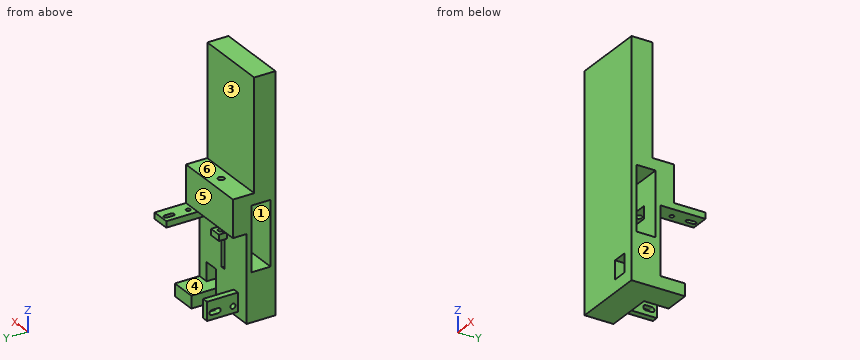
```python
from build123d import *

# Parameters (mm, degrees)
SKETCH1_W               = 60
SKETCH1_H               = 70
BOSS_EXTRUDE1_DEPTH     = 23.5
SHELL1_T                = -9
SKETCH2_W               = 10
SKETCH2_H               = 5
BOSS_EXTRUDE2_DEPTH     = 6.5
SKETCH5_W               = 60
SKETCH5_H               = 30
BOSS_EXTRUDE3_DEPTH     = 11
CUT_EXTRUDE1_DEPTH      = 83.554527435
CUT_EXTRUDE1_DEPTH_BACK = 83.554527435
SKETCH3_R               = 2.5
SKETCH4_W               = 30
SKETCH4_H               = 10
CUT_EXTRUDE2_DEPTH      = 10
SKETCH6_W               = 15
SKETCH6_H               = 5
BOSS_EXTRUDE4_DEPTH     = 36.5
SKETCH8_R               = 1.75
CUT_EXTRUDE3_DEPTH      = 10
SKETCH9_W               = 60
SKETCH9_H               = 23.5
BOSS_EXTRUDE5_DEPTH     = 30
CUT_EXTRUDE4_DEPTH      = 123.197585901
CUT_EXTRUDE4_DEPTH_BACK = 123.197585901
SKETCH11_W              = 12
SKETCH11_H              = 15
SKETCH12_W              = 5
SKETCH12_H              = 15
BOSS_EXTRUDE7_DEPTH     = 25
SKETCH13_R              = 2
CUT_EXTRUDE5_DEPTH      = 25
SKETCH14_W              = 21
SKETCH14_H              = 10
BOSS_EXTRUDE8_DEPTH     = 20
SKETCH15_W              = 60
SKETCH15_H              = 17.25
BOSS_EXTRUDE9_DEPTH     = 90
CUT_EXTRUDE6_DEPTH      = 132.148770486
CUT_EXTRUDE6_DEPTH_BACK = 132.148770486
SKETCH16_W              = 52
SKETCH16_H              = 15.5


with BuildPart() as part:
    # Sketch1 → Boss-Extrude1 (new body)
    with BuildSketch(Plane(origin=(0, 0, 0), x_dir=(1, 0, 0), z_dir=(0, 1, 0))):
        with Locations((-30, 35)):
            Rectangle(SKETCH1_W, SKETCH1_H)
    extrude(amount=BOSS_EXTRUDE1_DEPTH)

    # Shell1
    shell1_openings = [part.faces().sort_by_distance(p)[0] for p in [
        (-60, 11.75, -35),
        (0, 11.75, -35),
    ]]
    offset(amount=SHELL1_T, openings=shell1_openings, kind=Kind.INTERSECTION)

    # Sketch2 → Boss-Extrude2 (add)
    with BuildSketch(Plane(origin=(0, 23.5, 0), x_dir=(1, 0, 0), z_dir=(0, 1, 0))):
        with Locations((-30, 42.5)):
            Rectangle(SKETCH2_W, SKETCH2_H)
        with Locations((-30, 27.5)):
            Rectangle(SKETCH2_W, SKETCH2_H)
    extrude(amount=BOSS_EXTRUDE2_DEPTH)

    # Sketch5 → Boss-Extrude3 (add)
    with BuildSketch(Plane(origin=(0, 23.5, 0), x_dir=(1, 0, 0), z_dir=(0, 1, 0))):
        with Locations((-30, 15)):
            Rectangle(SKETCH5_W, SKETCH5_H)
    extrude(amount=BOSS_EXTRUDE3_DEPTH)

    # Sketch3 → Cut-Extrude1 (cut, two sides: drawn at the far end of the back side and taken through both)
    with BuildSketch(Plane(origin=(0, 0, -45), x_dir=(-1, 0, 0), z_dir=(0, 0, -1)).offset(-CUT_EXTRUDE1_DEPTH_BACK)):
        with Locations((30, 25)):
            Circle(SKETCH3_R)
    extrude(amount=CUT_EXTRUDE1_DEPTH + CUT_EXTRUDE1_DEPTH_BACK, mode=Mode.SUBTRACT)

    # Sketch4 → Cut-Extrude2 (cut)
    with BuildSketch(Plane(origin=(0, 23.5, 0), x_dir=(1, 0, 0), z_dir=(0, 1, 0))):
        with Locations((-30, 35)):
            Rectangle(SKETCH4_W, SKETCH4_H)
    extrude(amount=-CUT_EXTRUDE2_DEPTH, mode=Mode.SUBTRACT)

    # Sketch6 → Boss-Extrude4 (add)
    with BuildSketch(Plane(origin=(0, 23.5, 0), x_dir=(1, 0, 0), z_dir=(0, 1, 0))):
        with Locations((-7.5, 32.5)):
            Rectangle(SKETCH6_W, SKETCH6_H)
    extrude(amount=BOSS_EXTRUDE4_DEPTH)

    # Sketch8 → Cut-Extrude3 (cut)
    with BuildSketch(Plane(origin=(0, 0, -35), x_dir=(-1, 0, 0), z_dir=(0, 0, -1))):
        with Locations((9.05, 38.5)):
            Circle(SKETCH8_R)
        with BuildLine():
            Line((7.3, 56.5), (7.3, 51.5))
            ThreePointArc((7.3, 51.5), (9.05, 49.75), (10.8, 51.5))
            Line((10.8, 51.5), (10.8, 56.5))
            ThreePointArc((10.8, 56.5), (9.05, 58.25), (7.3, 56.5))
        make_face()
    extrude(amount=-CUT_EXTRUDE3_DEPTH, mode=Mode.SUBTRACT)

    # Sketch9 → Boss-Extrude5 (add)
    with BuildSketch(Plane(origin=(0, 0, -70), x_dir=(-1, 0, 0), z_dir=(0, 0, -1))):
        with Locations((30, 11.75)):
            Rectangle(SKETCH9_W, SKETCH9_H)
    extrude(amount=BOSS_EXTRUDE5_DEPTH)

    # Sketch11 → Cut-Extrude4 (cut, two sides: drawn at the far end of the back side and taken through both)
    with BuildSketch(Plane(origin=(0, 23.5, 0), x_dir=(1, 0, 0), z_dir=(0, 1, 0)).offset(-CUT_EXTRUDE4_DEPTH_BACK)):
        with Locations((-15, 82.5)):
            Rectangle(SKETCH11_W, SKETCH11_H)
    extrude(amount=CUT_EXTRUDE4_DEPTH + CUT_EXTRUDE4_DEPTH_BACK, mode=Mode.SUBTRACT)

    # Sketch12 → Boss-Extrude7 (add)
    with BuildSketch(Plane(origin=(0, 23.5, 0), x_dir=(1, 0, 0), z_dir=(0, 1, 0))):
        with Locations((-46.5, 88)):
            Rectangle(SKETCH12_W, SKETCH12_H)
    extrude(amount=BOSS_EXTRUDE7_DEPTH)

    # Sketch13 → Cut-Extrude5 (cut)
    with BuildSketch(Plane.ZY.offset(49)):
        with Locations((-90, 27.5)):
            Circle(SKETCH13_R)
        with BuildLine():
            Line((-88, 44.5), (-88, 39.5))
            ThreePointArc((-88, 39.5), (-90, 37.5), (-92, 39.5))
            Line((-92, 39.5), (-92, 44.5))
            ThreePointArc((-92, 44.5), (-90, 46.5), (-88, 44.5))
        make_face()
    extrude(amount=-CUT_EXTRUDE5_DEPTH, mode=Mode.SUBTRACT)

    # Sketch14 → Boss-Extrude8 (add)
    with BuildSketch(Plane(origin=(0, 23.5, 0), x_dir=(1, 0, 0), z_dir=(0, 1, 0))):
        with Locations((-10.5, 95)):
            Rectangle(SKETCH14_W, SKETCH14_H)
    extrude(amount=BOSS_EXTRUDE8_DEPTH)

    # Sketch15 → Boss-Extrude9 (add)
    with BuildSketch(Plane.XY):
        with Locations((-30, 8.625)):
            Rectangle(SKETCH15_W, SKETCH15_H)
    extrude(amount=BOSS_EXTRUDE9_DEPTH)

    # Sketch16 → Cut-Extrude6 (cut, two sides: drawn at the far end of the back side and taken through both)
    with BuildSketch(Plane(origin=(0, 0, 0), x_dir=(0, 0, -1), z_dir=(1, 0, 0)).offset(-CUT_EXTRUDE6_DEPTH_BACK)):
        with Locations((35, 11.75)):
            Rectangle(SKETCH16_W, SKETCH16_H)
    extrude(amount=CUT_EXTRUDE6_DEPTH + CUT_EXTRUDE6_DEPTH_BACK, mode=Mode.SUBTRACT)


solid = part.part
```
Here's how the part is built. I have some questions about the finished solid (model axes, mm). Face numbers are marked on the shaded views. A direction names the side the tool comes from. Give positions to 0.01 mm unless a question says otherwise; leave off trailing zeros. Write each loop counter-clockwise with the first axis right and the second up, starting at its lowest first coordinate (ties: lowest second). Pieces come first, ordered by that corner, then holes. Notation, with made-up numbers: (20, 40.5) -> (76, 40.5) arc R25 ccw to (76, 79.5) -> close; hole circle Ø7 at (55, 20). An arc over 180 degrees is marked (long way). Use one line per item in the form item = value.
1) Suppose I cut it at D-D (z = 71). Please give me the cut outline in (x, y), and give its area (4 significant figures).
Verdict:
outline = (-60, 0) -> (0, 0) -> (0, 17.25) -> (-60, 17.25) -> close
area = 1,035 mm2
2) On a 3-axis mill with a long thin cutter (end or side, diameter ignored), from which of +Z, -Z, +X, -X, +Y, -Y can I reach the whole of each face in a straight line? I mean the marked faces 1, 2 and 3. Say none if no direction works.
Verdict:
face_1 = +X, -X
face_2 = +Z, -Z, +X, +Y, -Y
face_3 = +Z, +X, -X, +Y
3) Suppose I cut it at C-C (x = -41). Please give me the cut outline in (y, z).
Verdict:
outline = (0, -100) -> (23.5, -100) -> (23.5, -40) -> (19.5, -40) -> (19.5, -61) -> (4, -61) -> (4, -9) -> (19.5, -9) -> (19.5, -30) -> (34.5, -30) -> (34.5, 0) -> (17.25, 0) -> (17.25, 90) -> (0, 90) -> close
4) Suppose I cut it at B-B (z = -47.5). Please give me the cut outline in (x, y), and give its area (3 significant figures).
Verdict:
outline = (-60, 0) -> (0, 0) -> (0, 4) -> (-60, 4) -> close; (-60, 19.5) -> (0, 19.5) -> (0, 23.5) -> (-28, 23.5) arc R2.5 cw to (-32, 23.5) -> (-60, 23.5) -> close
area = 477 mm2
5) I'm going to push flat-ended pins straight in: pin 1 (12 mm diameter, centred on x = -46, z = 32, fed in from +Y); pin 2 (9 mm diameter, centred on x = -31, z = -10, fed in from +Y); pin 3 (1.5 mm diameter, centred on x = -45.5, y = 42.5, fed in from +Z). Where does each tip first touch, or does it pass through?
Verdict:
pin_1 = 17.25
pin_2 = 34.5
pin_3 = -80.5
6) We'd pull the mould along Z, two halves only. Please class the marked faces 4, 5 and 6: +Z half, -Z half, draft (parallel to the pull), parting line (faces both ways), or undercut.
Verdict:
face_4 = undercut
face_5 = draft
face_6 = +Z half
7) Suppose I cut it at A-A (x = -30). Please give me the cut outline in (y, z).
Verdict:
outline = (0, -100) -> (23.5, -100) -> (23.5, -70) -> (22.5, -70) -> (22.5, -40) -> (19.5, -40) -> (19.5, -61) -> (4, -61) -> (4, -9) -> (19.5, -9) -> (19.5, -30) -> (22.5, -30) -> (22.5, 0) -> (17.25, 0) -> (17.25, 90) -> (0, 90) -> close; (27.5, -45) -> (30, -45) -> (30, -40) -> (27.5, -40) -> close; (27.5, -30) -> (34.5, -30) -> (34.5, 0) -> (27.5, 0) -> close
8) If I drill on L1, parallel to Y at x = -47.7, z = -90; L2, parallel to Y at x = -30, z = -47; L3, parallel to Y at x = -23, z = -14, over which ranges is the centre line in solid material (lowest first)? Write a range as [from, to].
Verdict:
L1 = [0, 25.5], [29.5, 37.5], [46.5, 48.5]
L2 = [0, 4], [19.5, 22.5]
L3 = [0, 4], [19.5, 34.5]
